For this review, take the finished solid that the model builds, in its own axes (mm). Face numbers are marked on the shaded views. A direction names the side the tool comes from. Coordinates: 2 decimals unless noted, no trailing zeros. Loops run counter-clockwise (first coordinate to the right, second up) from the corner with the lowest first, then second, coordinate; pieces in that order, holes last. Notation, with made-up numbers: M 59,-40 L 100,-40 A23 cw 100,-6 Z; hole C 84.25,-28.75 d10. An arc over 180 degrees is marked long. Use one line per item in the form item = value.
```python
from build123d import *

# Parameters (mm, degrees)
ESQUISSE1_R        = 11
ESQUISSE1_R_2      = 4
ESQUISSE1_R_3      = 1.65
BOSS_EXTRU_1_DEPTH = 2
ESQUISSE2_R        = 6
ESQUISSE2_R_2      = 4
BOSS_EXTRU_2_DEPTH = 7
CHANFREIN1_SIZE    = 0.5


with BuildPart() as part:
    # Esquisse1 → Boss.-Extru.1 (new body)
    with BuildSketch(Plane.XY):
        with Locations((65.66793974, 39.535817655)):
            Circle(ESQUISSE1_R)
        with Locations((65.66793974, 39.535817655)):
            Circle(ESQUISSE1_R_2, mode=Mode.SUBTRACT)
        with Locations((65.66793974, 48.035817655)):
            Circle(ESQUISSE1_R_3, mode=Mode.SUBTRACT)
        with Locations((74.16793974, 39.535817655)):
            Circle(ESQUISSE1_R_3, mode=Mode.SUBTRACT)
        with Locations((65.66793974, 31.035817655)):
            Circle(ESQUISSE1_R_3, mode=Mode.SUBTRACT)
        with Locations((57.16793974, 39.535817655)):
            Circle(ESQUISSE1_R_3, mode=Mode.SUBTRACT)
    extrude(amount=BOSS_EXTRU_1_DEPTH)

    # Esquisse2 → Boss.-Extru.2 (add)
    with BuildSketch(Plane.XY.offset(2)):
        with Locations((65.66793974, 39.535817655)):
            Circle(ESQUISSE2_R)
        with Locations((65.66793974, 39.535817655)):
            Circle(ESQUISSE2_R_2, mode=Mode.SUBTRACT)
    extrude(amount=BOSS_EXTRU_2_DEPTH)

    # Chanfrein1
    chanfrein1_edges = [part.edges().sort_by_distance(p)[0] for p in [
        (54.66793974, 39.535817655, 0),
        (59.66793974, 39.535817655, 9),
        (61.66793974, 39.535817655, 9),
        (54.66793974, 39.535817655, 2),
    ]]
    chamfer(chanfrein1_edges, length=CHANFREIN1_SIZE)


solid = part.part
```
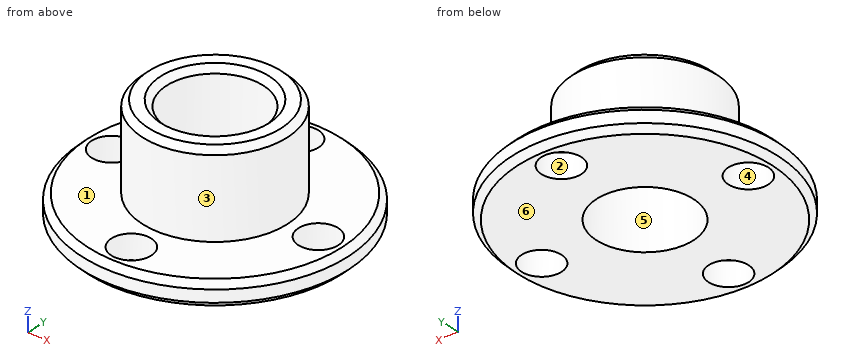
1. Draft analysis for pull direction X (two halves, no side actions). For the marked faces 3, 4, 5 and 6, state which applies: +X half, -X half, draft (parallel to the pull), parting line (faces both ways), or undercut.
Computed values:
face_3 = parting line
face_4 = undercut
face_5 = undercut
face_6 = draft
2. For pin 1 Ø2 at (y, z) = (37.5, 6) entering from -X; pin 2 Ø1.5 at (x, z) = (65, 3) entering from +Y; pin 3 Ø5.5 at (x, y) = (57.17, 39.54) entering from +Z, all flat-tipped, find the tip position at first contact; note any pin that passes through.
Computed values:
pin_1 = 59.76
pin_2 = 45.54
pin_3 = 8.75
3. Consider section B-B on z = 5.25. Write out the cut boundary in (x, y).
Computed values:
outline = C 65.67,39.54 d12; hole C 65.67,39.54 d8
4. Wall thickness on line 1 along Y through (x, z) = (65.75, 6); line 2 along X through (y, z) = (40.75, 6.25); line 3 along Y through (x, z) = (68.75, 0.75): over which ranges is each line inside the solid? List them lowest first. Write a range as from..to.
Computed values:
line_1 = 33.54..35.54, 43.53..45.54
line_2 = 59.79..61.86, 69.48..71.54
line_3 = 28.98..36.99, 42.09..50.1
5. Tool access review of the marked faces 1 and 2: name each direction out of +Z, -Z, +X, -X, +Y, -Y from which nothing blocks a thin tool from reaching the whole face with its end or side.
Computed values:
face_1 = +Z
face_2 = +Z, -Z
6. Consider section A-A on z = 1. Write out the cut boundary in (x, y), plus the area to 3 significant figures.
Computed values:
outline = C 65.67,39.54 d22; hole C 57.17,39.54 d3.3; hole C 65.67,39.54 d8; hole C 65.67,31.04 d3.3; hole C 65.67,48.04 d3.3; hole C 74.17,39.54 d3.3
area = 296 mm2
